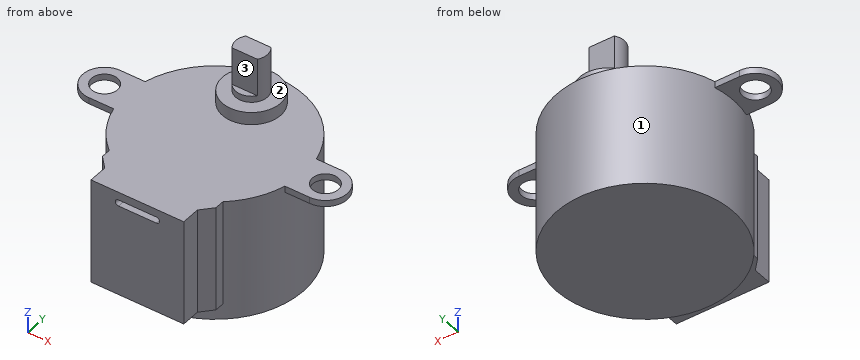
from build123d import *

# Parameters (mm, degrees)
SKETCH1_R           = 14
BOSS_EXTRUDE1_DEPTH = 19.3
BOSS_EXTRUDE2_START = -16.8
BOSS_EXTRUDE2_DEPTH = 16.8
CUT_EXTRUDE1_DEPTH  = 2
BOSS_EXTRUDE3_START = -1
SKETCH5_R           = 2.05
BOSS_EXTRUDE3_DEPTH = 1
SKETCH6_R           = 4.6
BOSS_EXTRUDE4_DEPTH = 2
SKETCH7_R           = 2.5
BOSS_EXTRUDE5_DEPTH = 7
CUT_EXTRUDE2_START  = -6
CUT_EXTRUDE2_DEPTH  = 6


with BuildPart() as part:
    # Sketch1 → Boss-Extrude1 (new body)
    with BuildSketch(Plane.XY):
        Circle(SKETCH1_R)
    extrude(amount=BOSS_EXTRUDE1_DEPTH)

    # Sketch2 → Boss-Extrude2 (add)
    with BuildSketch(Plane.XY.offset(19.3).offset(BOSS_EXTRUDE2_START)):
        with BuildLine():
            Line((-7.35, -17), (7.35, -17))
            Line((7.35, -17), (7.35, -14))
            Line((7.35, -14), (9, -12.223805295))
            Line((9, -12.223805295), (9, -10.723805295))
            ThreePointArc((9, -10.723805295), (0, -14), (-9, -10.723805295))
            Line((-9, -10.723805295), (-9, -12.223805295))
            Line((-9, -12.223805295), (-7.35, -14))
            Line((-7.35, -14), (-7.35, -17))
        make_face()
    extrude(amount=BOSS_EXTRUDE2_DEPTH)

    # Sketch4 → Cut-Extrude1 (cut)
    with BuildSketch(Plane.XZ.offset(17)):
        with BuildLine():
            Line((-3, 18.05), (3, 18.05))
            ThreePointArc((3, 18.05), (3.5, 17.55), (3, 17.05))
            Line((3, 17.05), (-3, 17.05))
            ThreePointArc((-3, 17.05), (-3.5, 17.55), (-3, 18.05))
        make_face()
    extrude(amount=-CUT_EXTRUDE1_DEPTH, mode=Mode.SUBTRACT)

    # Sketch5 → Boss-Extrude3 (add)
    # profile 1 of 2: a face of its own
    with BuildSketch(Plane.XY.offset(19.3).offset(BOSS_EXTRUDE3_START)):
        with BuildLine():
            Line((-17.5, 3.45), (-13.568253388, 3.45))
            ThreePointArc((-13.568253388, 3.45), (-14, 0), (-13.568253388, -3.45))
            Line((-13.568253388, -3.45), (-17.5, -3.45))
            ThreePointArc((-17.5, -3.45), (-20.95, 0), (-17.5, 3.45))
        make_face()
        with Locations((-17.5, 0)):
            Circle(SKETCH5_R, mode=Mode.SUBTRACT)
    # profile 2 of 2: a face of its own
    with BuildSketch(Plane.XY.offset(19.3).offset(BOSS_EXTRUDE3_START)):
        with BuildLine():
            Line((17.5, -3.45), (13.568253388, -3.45))
            ThreePointArc((13.568253388, -3.45), (14, 0), (13.568253388, 3.45))
            Line((13.568253388, 3.45), (17.5, 3.45))
            ThreePointArc((17.5, 3.45), (20.95, 0), (17.5, -3.45))
        make_face()
        with Locations(Location((17.5, 0, 0), (0, 0, 180))):
            Circle(SKETCH5_R, mode=Mode.SUBTRACT)
    extrude(amount=BOSS_EXTRUDE3_DEPTH)

    # Sketch6 → Boss-Extrude4 (add)
    with BuildSketch(Plane.XY.offset(19.3)):
        with Locations((0, 8)):
            Circle(SKETCH6_R)
    extrude(amount=BOSS_EXTRUDE4_DEPTH)

    # Sketch7 → Boss-Extrude5 (add)
    with BuildSketch(Plane.XY.offset(21.3)):
        with Locations((0, 8)):
            Circle(SKETCH7_R)
    extrude(amount=BOSS_EXTRUDE5_DEPTH)

    # Sketch8 → Cut-Extrude2 (cut)
    with BuildSketch(Plane.XY.offset(28.3).offset(CUT_EXTRUDE2_START)):
        with BuildLine():
            ThreePointArc((2, 9.5), (0, 10.5), (-2, 9.5))
            Line((-2, 9.5), (2, 9.5))
        make_face()
        with BuildLine():
            Line((2, 6.5), (-2, 6.5))
            ThreePointArc((-2, 6.5), (0, 5.5), (2, 6.5))
        make_face()
    extrude(amount=CUT_EXTRUDE2_DEPTH, mode=Mode.SUBTRACT)


solid = part.part
Design review of the part built by this model. Coordinates are the model's own, in mm. Face numbers are marked on the shaded views. A direction names the side the tool comes from. Coordinates: 2 decimals unless noted, no trailing zeros. Loops run counter-clockwise (first coordinate to the right, second up) from the corner with the lowest first, then second, coordinate; pieces in that order, holes last. Notation, with made-up numbers: (25.25, -19) - (37.25, -19) arc R7 ccw to (37.25, -9) - close; hole circle Ø9 at (35.5, 60.25). An arc over 180 degrees is marked (long way). Use CSV: the item, a comma, the result in double quotes. Start each with the question number.
1. Add section B-B on z = 17.55. Give the boundary of the cut face in (x, y).
2. Add section A-A on y = 0. Give the boundary of the cut face in (x, z).
3. Clearance check with flat-ended pins moving along their axes: pin 1 (3.5 mm diameter, centred on y = -15, z = 7, fed in from -X); pin 2 (3.5 mm diameter, centred on x = 18, y = 1.5, fed in from -Z); pin 3 (3 mm diameter, centred on x = -0.5, z = 26.5, fed in from +Y); pin 4 (1.1 mm diameter, centred on x = -1, z = 17.5, fed in from -Y). State where each tip first meets the part, or that it passes through.
4. Add section D-D on z = 12.25. Give the boundary of the cut face in (x, y).
5. For the marked faces 1, 2 and 3, list the 3-axis set-ups (+Z, -Z, +X, -X, +Y, -Y) from which the entire face can be reached by the end or side of a thin tool; tool diameter is ignored.
6. Add section C-C on x = 0. Give the boundary of the cut face in (y, z).
7. To check wall thickness, follow probe 1 along Y at (x, z) = (17.5, 19); probe 2 along Z at (x, y) = (5, -2.5); probe 3 along X at (y, z) = (11.5, 18.5). State the ranges of each line that lie inside material, in increasing order.
Resolved:
1,outline,"(-9, -12.22) - (-7.35, -14) - (-7.35, -17) - (-3.5, -17) - (-3.5, -15) - (3.5, -15) - (3.5, -17) - (7.35, -17) - (7.35, -14) - (9, -12.22) - (9, -10.72) arc R14 ccw (long way) to (-9, -10.72) - close"
2,outline,"(-20.95, 18.3) - (-19.55, 18.3) - (-19.55, 19.3) - (-20.95, 19.3) - close; (-15.45, 18.3) - (-14, 18.3) - (-14, 0) - (14, 0) - (14, 18.3) - (15.45, 18.3) - (15.45, 19.3) - (-15.45, 19.3) - close; (19.55, 18.3) - (20.95, 18.3) - (20.95, 19.3) - (19.55, 19.3) - close"
3,pin 1,"x = -8.05"
3,pin 2,"z = 18.3"
3,pin 3,"y = 9.5"
3,pin 4,"y = -17"
4,outline,"(-9, -12.22) - (-7.35, -14) - (-7.35, -17) - (7.35, -17) - (7.35, -14) - (9, -12.22) - (9, -10.72) arc R14 ccw (long way) to (-9, -10.72) - close"
5,face 1,"-Z"
5,face 2,"+Z"
5,face 3,"+Z, +X, -X, -Y"
6,outline,"(-17, 2.5) - (-14, 2.5) - (-14, 0) - (14, 0) - (14, 19.3) - (12.6, 19.3) - (12.6, 21.3) - (10.5, 21.3) - (10.5, 22.3) - (9.5, 22.3) - (9.5, 28.3) - (6.5, 28.3) - (6.5, 22.3) - (5.5, 22.3) - (5.5, 21.3) - (3.4, 21.3) - (3.4, 19.3) - (-17, 19.3) - (-17, 18.05) - (-15, 18.05) - (-15, 17.05) - (-17, 17.05) - close"
7,probe 1,"-3.45 to -2.05, 2.05 to 3.45"
7,probe 2,"0 to 19.3"
7,probe 3,"-7.98 to 7.98"
